Can you work these out from the model? Positions are in its coordinate system, mm. A direction names the side the tool comes from. Give positions to 0.01 mm unless a question says otherwise; leave off trailing zeros. Loops run counter-clockwise (first coordinate to the right, second up) from the corner with the lowest first, then second, coordinate; pieces in that order, holes last. Notation, with made-up numbers: (66.5, -1.75) -> (115.5, -1.75) arc R13 ccw to (115.5, 2.25) -> close; hole circle Ø2 at (11, 34.25). An arc over 180 degrees is marked (long way). One line per question, with ' | ' between items.
from build123d import *

# Parameters (mm, degrees)
F0_R     = 15
F1_DEPTH = 3
F2_DEPTH = 3
F3_DEPTH = 3


with BuildPart() as f1:
    # F0 (on Front) → F1 (new body)
    with BuildSketch(Plane.XZ):
        with BuildLine():
            ThreePointArc((-34, 27.5), (-34.2928932188, 26.7928932188), (-35, 26.5))
            Line((-35, 26.5), (-35, -26.5))
            ThreePointArc((-35, -26.5), (-34.2928932188, -26.7928932188), (-34, -27.5))
            Line((-34, -27.5), (-25, -27.5))
            add(Edge.make_bspline(
                [(-25, -27.5), (-16.6666666667, -25.25), (0, -20.75), (16.6666666667, -25.25), (25, -27.5)],
                knots=[0, 0, 0, 0, 0.5, 1, 1, 1, 1], degree=3))
            Line((25, -27.5), (34, -27.5))
            ThreePointArc((34, -27.5), (34.2928932188, -26.7928932188), (35, -26.5))
            Line((35, -26.5), (35, 26.5))
            ThreePointArc((35, 26.5), (34.2928932188, 26.7928932188), (34, 27.5))
            Line((34, 27.5), (25, 27.5))
            add(Edge.make_bspline(
                [(-25, 27.5), (-16.6666666667, 25.25), (0, 20.75), (16.6666666667, 25.25), (25, 27.5)],
                knots=[0, 0, 0, 0, 0.5, 1, 1, 1, 1], degree=3))
            Line((-25, 27.5), (-34, 27.5))
        make_face()
        with BuildLine():
            ThreePointArc((-21.75, -17), (-22.7019029611, -19.2980970389), (-25, -20.25))
            ThreePointArc((-25, -20.25), (-28.25, -17), (-25, -13.75))
            ThreePointArc((-25, -13.75), (-22.7019029611, -14.7019029611), (-21.75, -17))
        make_face(mode=Mode.SUBTRACT)
        with BuildLine():
            ThreePointArc((25, -13.75), (27.2980970389, -14.7019029611), (28.25, -17))
            ThreePointArc((28.25, -17), (27.2980970389, -19.2980970389), (25, -20.25))
            ThreePointArc((25, -20.25), (21.75, -17), (25, -13.75))
        make_face(mode=Mode.SUBTRACT)
        with BuildLine():
            ThreePointArc((-25, 13.75), (-27.2980970389, 19.2980970389), (-21.75, 17))
            ThreePointArc((-21.75, 17), (-22.7019029611, 14.7019029611), (-25, 13.75))
        make_face(mode=Mode.SUBTRACT)
        Circle(F0_R, mode=Mode.SUBTRACT)
        with BuildLine():
            ThreePointArc((25, 13.75), (21.75, 17), (25, 20.25))
            ThreePointArc((25, 20.25), (27.2980970389, 19.2980970389), (28.25, 17))
            ThreePointArc((28.25, 17), (27.2980970389, 14.7019029611), (25, 13.75))
        make_face(mode=Mode.SUBTRACT)
    extrude(amount=F1_DEPTH)

    # F0 (on Front) → F2 (join)
    with BuildSketch(Plane.XZ):
        with BuildLine():
            Line((-35, -26.5), (-35, 26.5))
            ThreePointArc((-35, 26.5), (-35.6028912237, 26.7021766033), (-35.9620014479, 27.2269556553))
            add(Edge.make_bspline(
                [(-70, 7), (-72.688876213, 8.6044405487), (-81.8919167368, 14.0958541424), (-55.1711599351, 21.7740976852), (-35.9620014479, 27.2269556553)],
                knots=[0, 0, 0, 0, 0.2887611513, 0.9883238821, 0.9883238821, 0.9883238821, 0.9883238821], degree=3))
            Line((-70, 7), (-60, 7))
            ThreePointArc((-60, 7), (-53, 0), (-60, -7))
            Line((-60, -7), (-70, -7))
            add(Edge.make_bspline(
                [(-70, -7), (-72.688876213, -8.6044405487), (-81.8919167368, -14.0958541424), (-55.1711599351, -21.7740976852), (-35.9620014479, -27.2269556553)],
                knots=[0, 0, 0, 0, 0.2887611513, 0.9883238821, 0.9883238821, 0.9883238821, 0.9883238821], degree=3))
            ThreePointArc((-35.9620014479, -27.2269556553), (-35.6028912237, -26.7021766033), (-35, -26.5))
        make_face()
        with BuildLine():
            add(Edge.make_bspline(
                [(-42, -12), (-55.9479149703, -11.5083551498), (-83.6545328023, -10.5317349163), (-56.7348192901, -15.3750907079), (-43.0358354206, -17.8155008402)],
                knots=[0, 0, 0, 0, 0.497194072, 0.9876433983, 0.9876433983, 0.9876433983, 0.9876433983], degree=3))
            ThreePointArc((-42, -12), (-39.8786796564, -12.8786796564), (-39, -15))
            ThreePointArc((-39, -15), (-39.8786796564, -17.1213203436), (-42, -18))
            ThreePointArc((-42, -18), (-42.5260691396, -17.9535150686), (-43.0358354206, -17.8155008402))
        make_face(mode=Mode.SUBTRACT)
        with BuildLine():
            ThreePointArc((-39, 15), (-39.8786796564, 12.8786796564), (-42, 12))
            add(Edge.make_bspline(
                [(-42, 12), (-55.9479149703, 11.5083551498), (-83.6545328023, 10.5317349163), (-56.7348192901, 15.3750907079), (-43.0358354206, 17.8155008402)],
                knots=[0, 0, 0, 0, 0.497194072, 0.9876433983, 0.9876433983, 0.9876433983, 0.9876433983], degree=3))
            ThreePointArc((-43.0358354206, 17.8155008402), (-42.5260691396, 17.9535150686), (-42, 18))
            ThreePointArc((-42, 18), (-39.8786796564, 17.1213203436), (-39, 15))
        make_face(mode=Mode.SUBTRACT)
    extrude(amount=F2_DEPTH)

    # F0 (on Front) → F3 (join)
    with BuildSketch(Plane.XZ):
        with BuildLine():
            ThreePointArc((35.9620014479, 27.2269556553), (35.6028912237, 26.7021766033), (35, 26.5))
            Line((35, 26.5), (35, -26.5))
            ThreePointArc((35, -26.5), (35.6028912237, -26.7021766033), (35.9620014479, -27.2269556553))
            add(Edge.make_bspline(
                [(75, -12), (74.084843936, -16.3392264677), (55.1711599351, -21.7740976852), (35.9620014479, -27.2269556553)],
                knots=[0.2887611513, 0.2887611513, 0.2887611513, 0.2887611513, 0.9883238821, 0.9883238821, 0.9883238821, 0.9883238821], degree=3))
            Line((75, -12), (75, -11.3173106911))
            add(Edge.make_bspline(
                [(70, -7), (72.3428093254, -8.3979439668), (74.6856186508, -9.7958879337), (75, -11.3173106911)],
                knots=[0, 0, 0, 0, 0.2515966763, 0.2515966763, 0.2515966763, 0.2515966763], degree=3))
            Line((70, -7), (60, -7))
            ThreePointArc((60, -7), (53, 0), (60, 7))
            Line((60, 7), (70, 7))
            add(Edge.make_bspline(
                [(35.9620014479, 27.2269556553), (55.1711599351, 21.7740976852), (81.8919167368, 14.0958541424), (72.688876213, 8.6044405487), (70, 7)],
                knots=[0.0116761179, 0.0116761179, 0.0116761179, 0.0116761179, 0.7112388487, 1, 1, 1, 1], degree=3))
        make_face()
        with BuildLine():
            ThreePointArc((42, -18), (39, -15), (42, -12))
            add(Edge.make_bspline(
                [(42, -12), (55.9479149703, -11.5083551498), (83.6545328023, -10.5317349163), (56.7348192901, -15.3750907079), (43.0358354206, -17.8155008402)],
                knots=[0, 0, 0, 0, 0.497194072, 0.9876433983, 0.9876433983, 0.9876433983, 0.9876433983], degree=3))
            ThreePointArc((43.0358354206, -17.8155008402), (42.5260691396, -17.9535150686), (42, -18))
        make_face(mode=Mode.SUBTRACT)
        with BuildLine():
            add(Edge.make_bspline(
                [(43.0358354206, 17.8155008402), (56.7348192901, 15.3750907079), (83.6545328023, 10.5317349163), (55.9479149703, 11.5083551498), (42, 12)],
                knots=[0.0123566017, 0.0123566017, 0.0123566017, 0.0123566017, 0.502805928, 1, 1, 1, 1], degree=3))
            ThreePointArc((42, 12), (39, 15), (42, 18))
            ThreePointArc((42, 18), (42.5260691396, 17.9535150686), (43.0358354206, 17.8155008402))
        make_face(mode=Mode.SUBTRACT)
    extrude(amount=F3_DEPTH)


solid = f1.part
Q1. If we mould it in two halves opening along Z, with no side actions, what happens to faces 1 (the face through (17, 0, 0)), 2 (the face through (53, -1, 0)), 3 (the face through (-29, -1, 27.5))? For each: pulls with the +Z half, pulls with the -Z half, needs draft (parallel to the pull), parting line crosses it, or undercut.
Entries:
face 1: needs draft | face 2: undercut | face 3: pulls with the +Z half
Q2. If I drill on probe 1 along Z at (x, y) = (-25, -1.15); probe 2 along Z at (x, y) = (-60, -1.75); probe 3 along Z at (x, y) = (0, -2.1), over which ranges is the centre line in solid material (lowest first)? Write a range as from..to.
Entries:
probe 1: -27.5..-20.25, -13.75..13.75, 20.25..27.5 | probe 2: -20.01..-14.7, -11.46..-7, 7..11.46, 14.7..20.01 | probe 3: -23..-15, 15..23
Q3. If we section it at A-A (z = 0): Write out the boundary of the cut face in (x, y), plus the area to 3 significant figures.
Entries:
outline: (-53, -3) -> (-15, -3) -> (-15, 0) -> (-53, 0) -> close; (15, -3) -> (53, -3) -> (53, 0) -> (15, 0) -> close | area: 228 mm²
Q4. On a 3-axis mill with a long thin cutter (end or side, diameter ignored), from which of +Z, -Z, +X, -X, +Y, -Y can I reach the whole of each face in a straight line? I mean faces 4 (the face through (29, -1, -27.5)), 5 (the face through (-65, -1, -7)), 6 (the face through (65, -1, 7)). Say none if no direction works.
Entries:
face 4: -Z, +X, -X, +Y, -Y | face 5: -X, +Y, -Y | face 6: +X, +Y, -Y
Q5. If we section it at B-B (y = -2.4): State how many separate pieces and enclosed holes the cut face has, plus the area to 3 significant figures.
Entries:
separate pieces: 1 | enclosed holes: 9 | area: 5,040 mm²
Q6. For pin 1 Ø0.9 at (x, y) = (66, -1.5) entering from +Z; pin 2 Ø0.9 at (x, y) = (-65, -2) entering from +Z; pin 3 Ø0.9 at (x, y) = (-64.5, -1.5) entering from -Z, each with a flat end and sliding along its axis, tell me the tip position at first contact or that it passes through.
Entries:
pin 1: z = 18 | pin 2: z = 18.39 | pin 3: z = -18.57
